Geometry check sheet. Reference: drawing and pictorial views, mm from the part's lowest x, y, z. Give positions to 0.01 mm unless a question says otherwise; leave off trailing zeros. Write each loop counter-clockwise with the first axis right and the second up, starting at its lowest first coordinate (ties: lowest second). Pieces come first, ordered by that corner, then holes. Notation, with made-up numbers: M 36.25,20 L 89.25,20 A30 ccw 89.25,53 Z; hole C 68,2 d6. An arc over 180 degrees is marked long. Write item = value, one per line. Start each with the question number.
1) Go/stop test with flat-tipped pins: pin 1 (0.8 mm diameter, centred on y = 8, z = 2.5, fed in from +X); pin 2 (6 mm diameter, centred on x = 2.5, y = 3.5, fed in from +Z); pin 3 (0.5 mm diameter, centred on x = 12, z = 2.5, fed in from -Y). Record where each tip stops, or that it passes through.
2) Cross-section at B-B, the plane x = 20. Record the cut outline in (y, z).
3) Cross-section at A-A, the plane y = 13. Record the cut outline in (x, z).
4) Scan lines: line 1 along X through (y, z) = (2, 1.05); line 2 along Y through (x, z) = (20, 1.2); line 3 along Y through (x, z) = (2.5, 1.65). Record each from-to range of solid material in increasing order. Write a range as [from, to].
5) Cross-section at D-D, the plane y = 6.75. Record the cut outline in (x, z).
6) Cross-section at C-C, the plane z = 1.6. Record the cut outline in (x, y), plus the area to 3 significant figures.
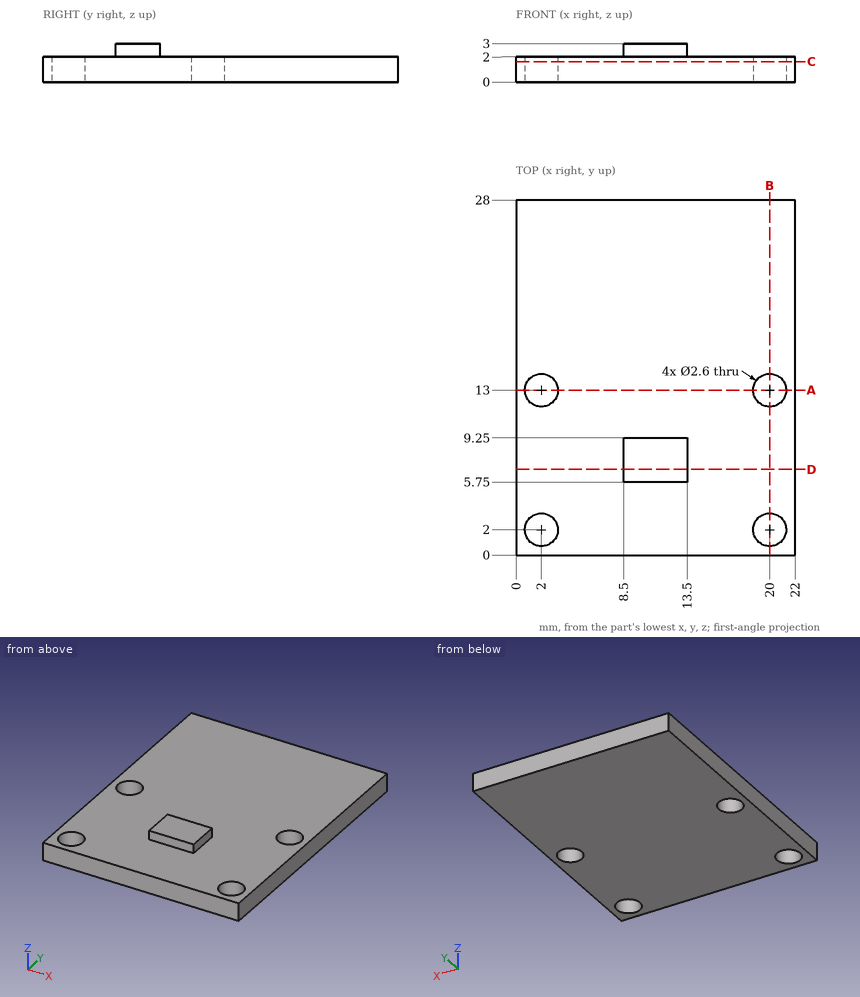
Reply:
q1.pin_1 = 13.5
q1.pin_2 = 2
q1.pin_3 = 5.75
q2.outline = M 0,0 L 0.7,0 L 0.7,2 L 0,2 Z; M 3.3,0 L 11.7,0 L 11.7,2 L 3.3,2 Z; M 14.3,0 L 28,0 L 28,2 L 14.3,2 Z
q3.outline = M 0,0 L 0.7,0 L 0.7,2 L 0,2 Z; M 3.3,0 L 18.7,0 L 18.7,2 L 3.3,2 Z; M 21.3,0 L 22,0 L 22,2 L 21.3,2 Z
q4.line_1 = [0, 0.7], [3.3, 18.7], [21.3, 22]
q4.line_2 = [0, 0.7], [3.3, 11.7], [14.3, 28]
q4.line_3 = [0, 0.8], [3.2, 11.8], [14.2, 28]
q5.outline = M 0,0 L 22,0 L 22,2 L 13.5,2 L 13.5,3 L 8.5,3 L 8.5,2 L 0,2 Z
q6.outline = M 0,0 L 22,0 L 22,28 L 0,28 Z; hole C 2,2 d2.6; hole C 2,13 d2.6; hole C 20,2 d2.6; hole C 20,13 d2.6
q6.area = 595 mm2
